Model file for the job. Use its own axes, mm. Face numbers are marked on the shaded views. A direction names the side the tool comes from. Coordinates: 2 decimals unless noted, no trailing zeros. Order: outer loops, then holes, each group sorted by start corner. A loop starts at its lowest first (then second) coordinate and runs counter-clockwise, first axis right, second up. Notation, with made-up numbers: (66, 36) -> (121, 36) arc R30 cw to (121, 64) -> close; hole circle Ø5 at (78.25, 13). An arc over 180 degrees is marked (long way). Return JSON: item names as keys, results as strings. Group by question number.
1) Cut at A-A (y = 12.75). Write the cut outline in (x, z).
2) Pull direction Z, two halves, no side cores. Call the marked faces 1, 2 and 3: +Z half, -Z half, draft (parallel to the pull), parting line (faces both ways), or undercut.
3) Cut at D-D (z = 0.5). State how many separate pieces and enclosed holes the cut face has, and give its area (3 significant figures).
4) Cut at B-B (x = 0). Write the cut outline in (y, z), and give its area (3 significant figures).
5) Probe line 1 (X direction, y = 1.6, z = 0); line 2 (Y direction, x = -5.25, z = 0); line 3 (Y direction, x = -4.7, z = 0). List the from-to ranges inside material, lowest first.
6) Which spindle directions (+Z, -Z, +X, -X, +Y, -Y) get a long thin tool onto all of the face, cutting with end or side? Do the marked faces 4, 5 and 6. Say none if no direction does.
7) Flat gauge pins, fed straight in: pin 1 (1.5 mm diameter, centred on y = 6, z = -3.5, fed in from -X); pin 2 (1 mm diameter, centred on y = 1.5, z = -4.5, fed in from -X); pin 3 (3 mm diameter, centred on y = 4, z = 2.5, fed in from +X); pin 4 (2.5 mm diameter, centred on y = 12, z = 0, fed in from -X). Where does each tip first touch, or does it go through?
8) Cut at C-C (y = 3). Write the cut outline in (x, z).
from build123d import *

# Parameters (mm, degrees)
SKETCH1_R               = 6
BOSS_EXTRUDE1_DEPTH     = 6
BOSS_EXTRUDE2_DEPTH     = 9
FILLET1_R               = 3
FILLET2_R               = 3
CUT_EXTRUDE2_DEPTH      = 18.233688096
CUT_EXTRUDE2_DEPTH_BACK = 18.233688096
SKETCH4_R               = 1.5
SKETCH5_R               = 5
CUT_EXTRUDE3_DEPTH      = 4


with BuildPart() as part:
    # Sketch1 → Boss-Extrude1 (new body)
    with BuildSketch(Plane(origin=(0, 0, 0), x_dir=(1, 0, 0), z_dir=(0, 1, 0))):
        with Locations(Location((0, 0, 0), (0, 0, 270))):
            Circle(SKETCH1_R)
    extrude(amount=BOSS_EXTRUDE1_DEPTH)

    # Sketch3 → Boss-Extrude2 (add)
    with BuildSketch(Plane(origin=(0, 6, 0), x_dir=(1, 0, 0), z_dir=(0, 1, 0))):
        with BuildLine():
            ThreePointArc((-4.512030676, 3.954943638), (-5.999972336, -0.01822004), (-4.487927828, -3.982273699))
            Line((-4.487927828, -3.982273699), (-3.362920912, -2.990110858))
            ThreePointArc((-3.362920912, -2.990110858), (-4.499963114, -0.01822004), (-3.38702376, 2.962780797))
            Line((-3.38702376, 2.962780797), (-4.512030676, 3.954943638))
        make_face()
        with BuildLine():
            Line((3.362920912, -2.990110858), (4.487927828, -3.982273699))
            ThreePointArc((4.487927828, -3.982273699), (5.609258729, -2.129839552), (6, 0))
            ThreePointArc((6, 0), (5.615700493, 2.112796245), (4.512030676, 3.954943638))
            Line((4.512030676, 3.954943638), (3.38702376, 2.962780797))
            ThreePointArc((3.38702376, 2.962780797), (4.499963114, -0.01822004), (3.362920912, -2.990110858))
        make_face()
    extrude(amount=BOSS_EXTRUDE2_DEPTH)

    # Fillet1
    # the kernel refuses this fillet: 3 mm, written as the material it takes off along each edge
    with BuildSketch(Plane(origin=(-2.262079088, 15, -1.970672851), x_dir=(0, -1, 0), z_dir=(0.7499999999999997, 0, 0.661437827766148)), Plane(origin=(10.137030676, 15, -8.915727346), x_dir=(0, -1, 0), z_dir=(-0.7499999999999997, 0, 0.661437827766148)), Plane(origin=(2.23797624, 15, 1.998002911), x_dir=(0, -1, 0), z_dir=(-0.7499999999999997, 0, -0.661437827766148)), Plane(origin=(-10.112927828, 15, 8.943057407), x_dir=(0, -1, 0), z_dir=(0.7499999999999997, 0, -0.661437827766148))) as fillet1_piece_1:
        with BuildLine():
            CenterArc((FILLET1_R, FILLET1_R), FILLET1_R, 180, 90)
            Line((0, FILLET1_R), (0, 0))
            Line((0, 0), (FILLET1_R, 0))
        make_face()
    extrude(amount=16.500009221, mode=Mode.SUBTRACT)

    # Fillet2
    # the kernel refuses this fillet: 3 mm, written as the material it adds along each edge
    with BuildSketch(Plane(origin=(-2.262079088, 6, -1.970672851), x_dir=(-0.661437827766148, 0, 0.7499999999999997), z_dir=(0.7499999999999997, 0, 0.661437827766148))) as fillet2_piece_1_section:
        with BuildLine():
            CenterArc((FILLET2_R, -FILLET2_R), FILLET2_R, 90, 90)
            Line((0, -FILLET2_R), (0, 0))
            Line((0, 0), (FILLET2_R, 0))
        make_face()
    fillet2_piece_1 = extrude(amount=16.500009221, mode=Mode.PRIVATE)
    fillet2_piece_1 = fillet2_piece_1 & Plane(origin=(0, 6.66993204, 0), x_dir=(0, 0, 1), z_dir=(0, -1, 0)) * Cylinder(6, 46, mode=Mode.PRIVATE)
    fillet2_piece_1 = fillet2_piece_1 - Plane(origin=(0, 6.66993204, 0), x_dir=(0.7526719465807102, 0, -0.6583957326945586), z_dir=(0, -1, 0)) * Cylinder(4.5, 46, mode=Mode.PRIVATE)
    add(fillet2_piece_1)
    with BuildSketch(Plane(origin=(10.137030676, 6, -8.915727346), x_dir=(-0.661437827766148, 0, -0.7499999999999998), z_dir=(-0.7499999999999997, 0, 0.661437827766148))) as fillet2_piece_2_section:
        with BuildLine():
            CenterArc((FILLET2_R, -FILLET2_R), FILLET2_R, 90, 90)
            Line((0, -FILLET2_R), (0, 0))
            Line((0, 0), (FILLET2_R, 0))
        make_face()
    fillet2_piece_2 = extrude(amount=16.500009221, mode=Mode.PRIVATE)
    fillet2_piece_2 = fillet2_piece_2 & Plane(origin=(0, 6.67033371, 0), x_dir=(0, 0, 1), z_dir=(0, -1, 0)) * Cylinder(6, 46, mode=Mode.PRIVATE)
    fillet2_piece_2 = fillet2_piece_2 - Plane(origin=(0, 6.67033371, 0), x_dir=(0.7526719465807102, 0, -0.6583957326945586), z_dir=(0, -1, 0)) * Cylinder(4.5, 46, mode=Mode.PRIVATE)
    add(fillet2_piece_2)
    with BuildSketch(Plane(origin=(-10.112927828, 6, 8.943057407), x_dir=(0.661437827766148, 0, 0.7499999999999998), z_dir=(0.7499999999999997, 0, -0.661437827766148))) as fillet2_piece_3_section:
        with BuildLine():
            CenterArc((FILLET2_R, -FILLET2_R), FILLET2_R, 90, 90)
            Line((0, -FILLET2_R), (0, 0))
            Line((0, 0), (FILLET2_R, 0))
        make_face()
    fillet2_piece_3 = extrude(amount=16.500009221, mode=Mode.PRIVATE)
    fillet2_piece_3 = fillet2_piece_3 & Plane(origin=(0, 6.669931793, 0), x_dir=(0, 0, 1), z_dir=(0, -1, 0)) * Cylinder(6, 46, mode=Mode.PRIVATE)
    fillet2_piece_3 = fillet2_piece_3 - Plane(origin=(0, 6.669931793, 0), x_dir=(-0.7473157581885724, 0, 0.6644690794634761), z_dir=(0, -1, 0)) * Cylinder(4.5, 46, mode=Mode.PRIVATE)
    add(fillet2_piece_3)
    with BuildSketch(Plane(origin=(2.23797624, 6, 1.998002911), x_dir=(0.661437827766148, 0, -0.7499999999999997), z_dir=(-0.7499999999999997, 0, -0.661437827766148))) as fillet2_piece_4_section:
        with BuildLine():
            CenterArc((FILLET2_R, -FILLET2_R), FILLET2_R, 90, 90)
            Line((0, -FILLET2_R), (0, 0))
            Line((0, 0), (FILLET2_R, 0))
        make_face()
    fillet2_piece_4 = extrude(amount=16.500009221, mode=Mode.PRIVATE)
    fillet2_piece_4 = fillet2_piece_4 & Plane(origin=(0, 6.670333879, 0), x_dir=(0, 0, 1), z_dir=(0, -1, 0)) * Cylinder(6, 46, mode=Mode.PRIVATE)
    fillet2_piece_4 = fillet2_piece_4 - Plane(origin=(0, 6.670333879, 0), x_dir=(-0.7473157581885724, 0, 0.6644690794634761), z_dir=(0, -1, 0)) * Cylinder(4.5, 46, mode=Mode.PRIVATE)
    add(fillet2_piece_4)

    # Sketch4 → Cut-Extrude2 (cut, two sides: drawn at the far end of the back side and taken through both)
    with BuildSketch(Plane(origin=(0, 0, 0), x_dir=(0, 0, -1), z_dir=(1, 0, 0)).offset(-CUT_EXTRUDE2_DEPTH_BACK)):
        with Locations((0, 12)):
            Circle(SKETCH4_R)
    extrude(amount=CUT_EXTRUDE2_DEPTH + CUT_EXTRUDE2_DEPTH_BACK, mode=Mode.SUBTRACT)

    # Sketch5 → Cut-Extrude3 (cut)
    with BuildSketch(Plane.XZ):
        with Locations(Location((0, 0, 0), (0, 0, 270))):
            Circle(SKETCH5_R)
    extrude(amount=-CUT_EXTRUDE3_DEPTH, mode=Mode.SUBTRACT)


solid = part.part
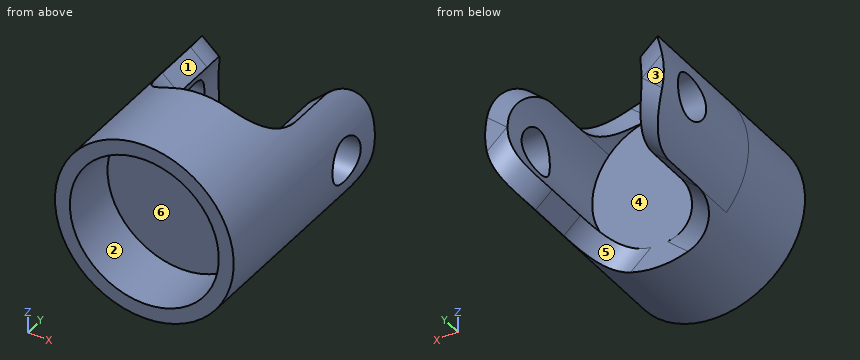
Answers below:
{
 "1": {"outline": "(-5.86, -1.3) arc R6 ccw to (-4.57, -3.88) -> (-3.45, -2.89) arc R4.5 cw to (-4.31, -1.3) -> close; (-5.86, 1.3) -> (-4.31, 1.3) arc R4.5 cw to (-3.43, 2.92) -> (-4.55, 3.91) arc R6 ccw to start; (3.43, 2.92) arc R4.5 cw to (4.31, 1.3) -> (5.86, 1.3) arc R6 ccw to (4.55, 3.91) -> close; (3.45, -2.89) -> (4.57, -3.88) arc R6 ccw to (5.86, -1.3) -> (4.31, -1.3) arc R4.5 cw to start"},
 "2": {"face 1": "+Z half", "face 2": "undercut", "face 3": "draft"},
 "3": {"separate pieces": "3", "enclosed holes": "0", "area": "50.5 mm^2"},
 "4": {"outline": "(0, -6) -> (6, -6) -> (6, 6) -> (0, 6) -> (0, 5) -> (4, 5) -> (4, -5) -> (0, -5) -> close", "area": "32.0 mm^2"},
 "5": {"line 1": "x = -6 to -5, 5 to 6", "line 2": "y = 0 to 10.5, 13.5 to 15", "line 3": "y = 4 to 10.5, 13.5 to 15"},
 "6": {"face 4": "+Y", "face 5": "-Z, +Y", "face 6": "-Y"},
 "7": {"pin 1": "stops at x = -5.33", "pin 2": "stops at x = -4.47", "pin 3": "stops at x = 5.92", "pin 4": "passes through"},
 "8": {"outline": "circle Ø12 at (0, 0); hole circle Ø10 at (0, 0)"}
}
